Autodesk Inventor part; units mm, degrees
ref_plane "Work Plane1" through (0, 25, 0) normal (0, 1, 0) x (-1, 0, 0)
ref_plane "YZ Plane" through (0, 0, 0) normal (1, 0, 0) x (0, 1, 0)
ref_plane "XY Plane" through (0, 0, 0) normal (0, 0, 1) x (1, 0, 0)
sketch "Sketch1" plane through (0, 0, 0) normal (0, 0, 1) x (1, 0, 0)
  circle A0 centre (0, 0) radius 25
  line L0 (-14.5, 17.25) -> (14.5, 17.25)
  line L1 (14.5, 17.25) -> (14.5, -17.25)
  line L2 (14.5, -17.25) -> (-14.5, -17.25)
  line L3 (-14.5, -17.25) -> (-14.5, 17.25)
  dimension "d0" = 50
  dimension "d1" = 29
  dimension "d2" = 34.5
  dimension "d3" = 14.5
  dimension "d4" = 17.25
extrude "Extrusion1" add sketch "Sketch1" along normal blind 30 contours A0 | L0 L1 L2 L3
sketch "Sketch2" plane through (0, 0, 30) normal (0, 0, 1) x (1, 0, 0)
  circle A0 centre (0, 0) radius 25
  line L0 (-20, 15) -> (20, 15)
  line L1 (-20, -15) -> (20, -15)
  dimension "d14" = 30
  dimension "d15" = 15
extrude "Extrusion2" add sketch "Sketch2" along normal blind 15 contours A0 L1 L0
sketch "Sketch4" plane through (-20, 15, 30) normal (0, 1, 0) x (1, 0, 0)
  circle A0 centre (20, -90) radius 100
  line L0 (40, -15) -> (0, -15)
  line L1 (-5, 30) -> (-5, -15)
  point P0 (20, 30)
  dimension "d16" = 75
  dimension "d17" = 25
  dimension "d18" = 200
extrude "Extrusion4" cut sketch "Sketch4" along normal blind 10
mirror "Mirror1" about plane through (0, 0, 0) normal (0, 1, 0) of "Extrusion4"
sketch "Sketch5" plane through (0, 0, 0) normal (0, 0, -1) x (-1, 0, 0)
  line L0 (14.5, -17.25) -> (-14.5, -17.25)
  line L1 (-14.5, -17.25) -> (-14.5, 17.25)
  line L2 (-14.5, 17.25) -> (14.5, 17.25)
  line L3 (14.5, 17.25) -> (14.5, -17.25)
  point P0 (0, 0)
  dimension "d21" = 34.5
  dimension "d22" = 29
  dimension "d23" = 17.25
  dimension "d24" = 14.5
extrude "Extrusion5" cut sketch "Sketch5" against normal blind 17
ref_plane "Work Plane1" through (0, 25, 0) normal (0, 1, 0) x (-1, 0, 0)
sketch "Sketch6" plane through (0, 25, 0) normal (0, 1, 0) x (-1, 0, 0)
  circle A0 centre (-11, 10) radius 1.5
  circle A1 centre (11, 10) radius 1.5
  line L0 (25, 0) -> (-25, 0)
  line L1 (-14.5, 0) -> (-14.5, 17)
  point P0 (0, 0)
  point P1 (-14.5, 16.0568)
  dimension "d28" = 3
  dimension "d29" = 3
  dimension "d30" = 10
  dimension "d31" = 10
  dimension "d32" = 22
  dimension "d33" = 3.5
extrude "Extrusion6" cut sketch "Sketch6" against normal blind 50
sketch "Sketch7" plane through (0, 25, 0) normal (0, 1, 0) x (-1, 0, 0)
  circle A0 centre (-11, 10) radius 1.5
  circle A1 centre (-11, 10) radius 3
  circle A2 centre (11, 10) radius 1.5
  circle A3 centre (11, 10) radius 3
  point P0 (0, 0)
  dimension "d36" = 6
  dimension "d37" = 6
extrude "Extrusion7" cut sketch "Sketch7" against normal blind 5 contours A0 | A1 | A2 | A3
mirror "Mirror2" about plane through (0, 0, 0) normal (0, 1, 0) of "Extrusion7"
sketch "Sketch9" plane through (0, 0, 45) normal (0, 0, 1) x (1, 0, 0)
  line L0 (-14.5, 10) -> (14.5, 10)
  line L1 (14.5, 10) -> (14.5, -10)
  line L2 (14.5, -10) -> (-14.5, -10)
  line L3 (-14.5, -10) -> (-14.5, 10)
  line L4 (20, 15) -> (-20, 15)
  line L5 (-20, -15) -> (20, -15)
  point P0 (0, 0)
  dimension "d57" = 29
  dimension "d58" = 14.5
  dimension "d64" = 5
  dimension "d65" = 5
extrude "Extrusion9" cut sketch "Sketch9" against normal blind 40
chamfer "Chamfer1" distance 7.25 angle 45 2 edges at (0, 10, 17) (0, -10, 17)
sketch "Sketch10" plane through (-20, -15, 45) normal (0, -1, 0) x (1, 0, 0)
  circle A0 centre (18.0952, -5) radius 2.0666
  circle A1 centre (18.0952, -15) radius 2.0679
  line L0 (0, 0) -> (40, 0)
  line L1 (7.0094, -25) -> (36.1661, -25)
  arc A2 (0, -22.9796) -> (40, -22.9796) centre (20, 75) ccw
  point P0 (20, -45)
  point P1 (18.0952, -25)
  point P2 (32.5952, -28.9432)
  dimension "d66" = 15
  dimension "d67" = 5
extrude "Extrusion10" cut sketch "Sketch10" against normal blind 40
equation "\"d15\" = 0.5 * d14"
equation "\"d65\" = d64"
properties part number "RL_spider_leg_mount"
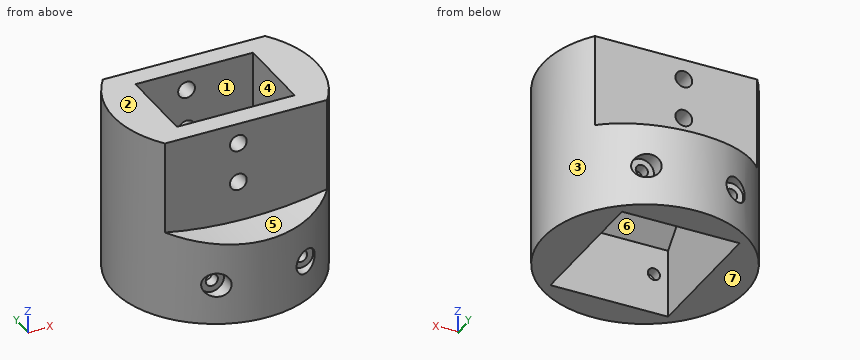
Design review of the part built by this model. Coordinates are the model's own, in mm. Face numbers are marked on the shaded views. A direction names the side the tool comes from. Round coordinates to 2 decimals unless told otherwise and drop trailing zeros. Write each loop counter-clockwise with the first axis right and the second up, starting at its lowest first coordinate (ties: lowest second). Pieces come first, ordered by that corner, then holes.
Item 1: For the marked faces 5, 6 and 7, list the 3-axis set-ups (+Z, -Z, +X, -X, +Y, -Y) from which the entire face can be reached by the end or side of a thin tool; tool diameter is ignored.
Item 2: Draft analysis for pull direction Y (two halves, no side actions). For the marked faces 1, 2, 3 and 4, state which applies: released by +Y, released by -Y, zero draft, split by the parting line, or undercut.
Item 3: Consider section A-A on y = 0. Give the boundary of the cut face in (x, z), and give its area (3 significant figures).
Item 4: For pin 1 Ø5 at (x, z) = (-11, 10) entering from +Y; pin 2 Ø2.5 at (x, z) = (-1.9, 40) entering from -Y; pin 3 Ø6.5 at (x, z) = (12.5, 11) entering from -Y; pin 4 Ø9.5 at (x, z) = (-11, 10) entering from -Y, all flat-tipped, find the tip position at first contact; note any pin that passes through.
Item 5: Consider section C-C on x = -11. Count the separate pieces of the cut face and the enclosed holes in it, and give its area (3 significant figures).
Item 6: Consider section B-B on z = 40. Give the boundary of the cut face in (x, y), and give its area (3 significant figures).
Item 7: Wall thickness on L1, parallel to Y at x = -9.5, z = 42; L2, parallel to X at y = -22.75, z = 10; L3, parallel to Z at x = -11, y = 18.7: over which ranges is each line inside the solid? List them lowest first.
Item 8: Consider section D-D on z = 29. Give the boundary of the cut face in (x, y), and give its area (3 significant figures).
Check values:
1. face 5: +Z, -Y
1. face 6: -Z
1. face 7: -Z, +X, -X, +Y, -Y
2. face 1: undercut
2. face 2: zero draft
2. face 3: split by the parting line
2. face 4: undercut
3. outline: (-25, 0) - (-14.5, 0) - (-14.5, 45) - (-25, 45) - close; (14.5, 0) - (25, 0) - (25, 45) - (14.5, 45) - close
3. area: 945 mm2
4. pin 1: stops at y = 20
4. pin 2: passes through
4. pin 3: stops at y = -23.02
4. pin 4: stops at y = -24.21
5. separate pieces: 4
5. enclosed holes: 0
5. area: 412 mm2
6. outline: (-20, -15) - (-3.97, -15) - (-3.97, -10) - (-14.5, -10) - (-14.5, 10) - (-3.97, 10) - (-3.97, 15) - (-20, 15) arc R25 ccw to start; (0.16, -15) - (20, -15) arc R25 ccw to (20, 15) - (0.16, 15) - (0.16, 10) - (14.5, 10) - (14.5, -10) - (0.16, -10) - close
6. area: 783 mm2
7. L1: y = -15 to -10, 10 to 15
7. L2: x = -8 to 8
7. L3: z = 0 to 8.5, 11.5 to 20.61
8. outline: (-20, -15) - (-3.71, -15) - (-3.71, -10) - (-14.5, -10) - (-14.5, 10) - (-3.71, 10) - (-3.71, 15) - (-20, 15) arc R25 ccw to start; (-0.09, -15) - (20, -15) arc R25 ccw to (20, 15) - (-0.09, 15) - (-0.09, 10) - (14.5, 10) - (14.5, -10) - (-0.09, -10) - close
8. area: 788 mm2
